from build123d import *

# Parameters (mm, degrees)
F1_DEPTH = 114.3
F2_R     = 1.5875
F3_DEPTH = 25.4
F4_SIZE  = 1.27
F5_R     = 3.175


with BuildPart() as f1:
    # F0 (on Right) → F1 (new body)
    with BuildSketch(Plane.YZ):
        Polygon((-69.0606392323, 6.6139034851), (-69.0606392323, 0), (70.6393607677, 40.6923843751), (70.6393607677, 47.3062878602), align=None)
    extrude(amount=F1_DEPTH)

    # F2 (on face) → F3 (cut)
    with BuildSketch(Plane(origin=(0, -7.177119146, 24.6395869914), x_dir=(1, 0, 0), z_dir=(0, -0.2796614495, 0.9600986791))):
        with BuildLine():
            Line((73.025, 71.525502), (41.275, 71.525502))
            ThreePointArc((41.275, 71.525502), (39.0299359698, 70.5955660302), (38.1, 68.350502))
            Line((38.1, 68.350502), (38.1, 62.000502))
            ThreePointArc((38.1, 62.000502), (39.0299359697, 59.7554379697), (41.275, 58.825502))
            Line((41.275, 58.825502), (73.025, 58.825502))
            ThreePointArc((73.025, 58.825502), (75.2700640303, 59.7554379697), (76.2, 62.000502))
            Line((76.2, 62.000502), (76.2, 68.350502))
            ThreePointArc((76.2, 68.350502), (75.2700640302, 70.5955660302), (73.025, 71.525502))
        make_face()
        with Locations((4.1148, 76.935702)):
            Circle(F2_R)
        with Locations((110.1852, 76.935702)):
            Circle(F2_R)
        with Locations((110.1852, -60.3405746722)):
            Circle(F2_R)
        with Locations((4.1148, -60.3405746722)):
            Circle(F2_R)
    extrude(amount=-F3_DEPTH, mode=Mode.SUBTRACT)

    # F4
    f4_edges = [f1.edges().sort_by_distance(p)[0] for p in [
        (108.5977, 66.688747, 46.155537),
        (108.5977, -65.110025, 7.764654),
        (2.5273, -65.110025, 7.764654),
        (2.5273, 66.688747, 46.155537),
        (57.15, 61.494421, 44.642513),
        (39.029936, 60.601591, 44.382445),
        (38.1, 55.397794, 42.866662),
        (39.029936, 50.193998, 41.350879),
        (57.15, 49.301168, 41.090812),
        (75.270064, 50.193998, 41.350879),
        (76.2, 55.397794, 42.866662),
        (75.270064, 60.601591, 44.382445),
        (57.15, 51.077018, 34.994186),
        (75.270064, 51.969848, 35.254253),
    ]]
    chamfer(f4_edges, length=F4_SIZE)

    # F5
    f5_edges = [f1.edges().sort_by_distance(p)[0] for p in [
        (114.3, -69.060639, 3.306952),
        (114.3, 70.639361, 43.999336),
        (0, -69.060639, 3.306952),
        (0, 70.639361, 43.999336),
    ]]
    fillet(f5_edges, radius=F5_R)


solid = f1.part
Verification items for the finished model (mm, model axes). A direction names the side the tool comes from. Round coordinates to 2 decimals unless told otherwise and drop trailing zeros. Write each loop counter-clockwise with the first axis right and the second up, starting at its lowest first coordinate (ties: lowest second). Pieces come first, ordered by that corner, then holes.
(1) Mould release check, pull along Y, two halves, no side actions. Record for faces 4 (the flat face through (56.215, 1.767, 27.245)), 5 (the flat face through (114.3, 0, 24)), 6 (the cylindrical face through (111.7, 68.2, 42.67)), 7 (the flat face through (56.35, -0.19, 20.06)): pulls with the +Y half, pulls with the -Y half, needs draft (parallel to the pull), parting line crosses it, or undercut.
Returned:
face 4: pulls with the -Y half
face 5: needs draft
face 6: undercut
face 7: pulls with the +Y half
(2) Access from +Z, -Z, +X, -X, +Y, -Y to the whole of each face (thin tool, end or side, straight path). Record for faces 1 (the flat face through (56.93, 50.18, 38.07)), 2 (the flat face through (56, 70.639, 44)), 3 (the cylindrical face through (75.295, 61.458, 41.353)).
Returned:
face 1: +Z
face 2: +Z, -Z, +X, -X, +Y
face 3: -Z
(3) Material ranges on line 1 (Z direction, x = 80, y = -56); line 2 (Z direction, x = 13, y = 13.5), recorded low to high.
Returned:
line 1: z = 3.8 to 10.42
line 2: z = 24.05 to 30.66
(4) Depth check by flat-ended pin: pin 1 Ø1 at (x, y) = (41, -1.5) entering from +Z; pin 2 Ø5 at (x, y) = (97, -37.5) entering from -Z; pin 3 Ø2 at (x, y) = (73, -21) entering from +Z. Enter the tip coordinate at first touch or a pass-through.
Returned:
pin 1: stops at z = 26.44
pin 2: stops at z = 8.46
pin 3: stops at z = 20.9
(5) Section check B-B (x = 25.5). Enter the section's corners in (y, z), plus the area to 3 significant figures.
Returned:
outline: (-69.06, 0) - (70.64, 40.69) - (70.64, 47.31) - (-69.06, 6.61) - close
area: 924 mm2
(6) Section check C-C (y = -34). Enter the section's corners in (x, z), plus the area to 3 significant figures.
Returned:
outline: (0, 10.21) - (114.3, 10.21) - (114.3, 16.83) - (0, 16.83) - close
area: 756 mm2
(7) Section check A-A (x = 46). Enter the section's corners in (y, z).
Returned:
outline: (-69.06, 0) - (49.86, 34.64) - (50.72, 36.21) - (49.66, 39.87) - (48.08, 40.74) - (-69.06, 6.61) - close; (61.85, 43.42) - (62.92, 39.77) - (64.49, 38.9) - (70.64, 40.69) - (70.64, 47.31) - (62.71, 45) - close
